The listing builds one solid part. Answer for the finished solid, in the listing's coordinates (mm). Face numbers are marked on the shaded views. A direction names the side the tool comes from. Coordinates: 2 decimals unless noted, no trailing zeros. Order: outer loops, then holes, each group sorted by start corner. A loop starts at its lowest first (then second) coordinate and runs counter-clockwise, first axis right, second up. Notation, with made-up numbers: (18, 43.5) -> (42, 43.5) arc R15 ccw to (42, 52.5) -> close; hole circle Ø1 at (41, -29.5). An arc over 180 degrees is marked (long way). Put each result on its own line as item: value. Start each with the question number.
```python
from build123d import *

# Parameters (mm, degrees)
SKETCH1_R           = 27
SKETCH1_R_2         = 8.8
BOSS_EXTRUDE1_DEPTH = 6.2
BOSS_EXTRUDE2_START = 2
SKETCH2_R           = 32.5
SKETCH2_R_2         = 8.8
BOSS_EXTRUDE2_DEPTH = 2
SKETCH3_W           = 5
SKETCH3_H           = 4.39677325
SKETCH3_W_2         = 4.39677325
SKETCH3_H_2         = 5
BOSS_EXTRUDE3_DEPTH = 6.2
BOSS_EXTRUDE4_DEPTH = 6.2


with BuildPart() as part:
    # Sketch1 → Boss-Extrude1 (new body)
    with BuildSketch(Plane(origin=(0, 0, 0), x_dir=(1, 0, 0), z_dir=(0, 1, 0))):
        with Locations(Location((0, 0, 0), (0, 0, 90))):
            Circle(SKETCH1_R)
        with Locations(Location((0, 0, 0), (0, 0, 90))):
            Circle(SKETCH1_R_2, mode=Mode.SUBTRACT)
        with BuildLine():
            Line((-17.5, -17.360083525), (-13.240365112, -13.134505385))
            ThreePointArc((-13.240365112, -13.134505385), (-17.20219229, -7.204656856), (-18.648686612, -0.221331548))
            Line((-18.648686612, -0.221331548), (-17.148571199, -0.221372599))
            ThreePointArc((-17.148571199, -0.221372599), (-15.815189186, -6.633422269), (-12.175456389, -12.07811085))
            Line((-12.175456389, -12.07811085), (-7.915821501, -7.85253271))
            ThreePointArc((-7.915821501, -7.85253271), (0, 11.15), (7.915821501, -7.85253271))
            Line((7.915821501, -7.85253271), (12.175456389, -12.07811085))
            ThreePointArc((12.175456389, -12.07811085), (15.815189186, -6.633422269), (17.148571199, -0.221372599))
            Line((17.148571199, -0.221372599), (18.648686612, -0.221331548))
            ThreePointArc((18.648686612, -0.221331548), (17.20219229, -7.204656856), (13.240365112, -13.134505385))
            Line((13.240365112, -13.134505385), (17.5, -17.360083525))
            ThreePointArc((17.5, -17.360083525), (0, 24.65), (-17.5, -17.360083525))
        make_face(mode=Mode.SUBTRACT)
    extrude(amount=BOSS_EXTRUDE1_DEPTH)

    # Sketch2 → Boss-Extrude2 (add)
    with BuildSketch(Plane.XZ.offset(BOSS_EXTRUDE2_START)):
        with Locations(Location((0, 0, 0), (0, 0, 270))):
            Circle(SKETCH2_R)
        with Locations(Location((0, 0, 0), (0, 0, 270))):
            Circle(SKETCH2_R_2, mode=Mode.SUBTRACT)
    extrude(amount=-BOSS_EXTRUDE2_DEPTH)

    # Sketch3 → Boss-Extrude3 (add)
    with BuildSketch(Plane(origin=(0, 0, 0), x_dir=(1, 0, 0), z_dir=(0, 1, 0))):
        with Locations((0, 27.601613375)):
            Rectangle(SKETCH3_W, SKETCH3_H)
        with Locations((27.601613375, 0)):
            Rectangle(SKETCH3_W_2, SKETCH3_H_2)
        with Locations((0, -27.601613375)):
            Rectangle(SKETCH3_W, SKETCH3_H)
        with Locations((-27.601613375, 0)):
            Rectangle(SKETCH3_W_2, SKETCH3_H_2)
    extrude(amount=BOSS_EXTRUDE3_DEPTH)

    # Sketch5 → Boss-Extrude4 (add)
    with BuildSketch(Plane(origin=(0, 0, 0), x_dir=(1, 0, 0), z_dir=(0, 1, 0))):
        with BuildLine():
            Line((-18.97760125, -15.731279376), (-13.203483223, -10.944886057))
            ThreePointArc((-13.203483223, -10.944886057), (-12.702113744, -11.522968647), (-12.175456389, -12.07811085))
            Line((-12.175456389, -12.07811085), (-17.733930638, -18.204578298))
            Line((-17.733930638, -18.204578298), (-18.97760125, -15.731279376))
        make_face()
    boss_extrude4 = extrude(amount=BOSS_EXTRUDE4_DEPTH)

    # Mirror2: Boss-Extrude4 across plane
    add(boss_extrude4.mirror(Plane(origin=(0, 0, 0), x_dir=(0, 0, 1), z_dir=(1, 0, 0))))


solid = part.part
```
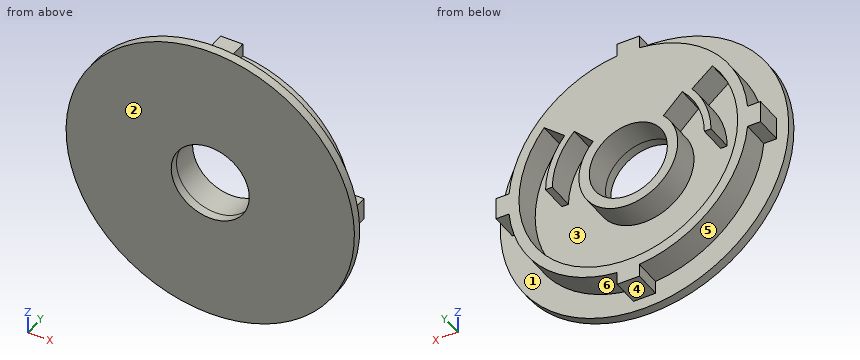
(1) The part is cut by section A-A on x = 0. Determine the outline of the cut face in (y, z), plus the area to 4 significant figures.
(2) Each of these flat-tipped pins is pushed along its axis until it touches: P1, Ø0.9, axis at y = 3.5, z = -28, coming from the +X side; P2, Ø1.5, axis at x = 1, y = 4, coming from the -Z side; P3, Ø1.5, axis at x = -1, y = 3, coming from the +Z side. Where does it stop, or does it pass through?
(3) The part is cut by section B-B on y = 1.5. Count the separate pieces of the cut face and the enclosed holes in it, plus the area to 3 significant figures.
(4) A tool of negligible diameter and unlimited length cuts with its end or side. For the marked faces 1 and 2, from which of +Z, -Z, +X, -X, +Y, -Y can it reach the whole face along a straight path? Write none if from no direction.
(5) For a pull along X with two mould halves and no side action, classify the marked faces 3, 4, 5 and 6 as released by +X, released by -X, zero draft, split by the parting line, or undercut.
(6) Find the intervals of material crossed by L1, parallel to Z at x = 0, y = 5; L2, parallel to X at y = 2, z = 0; L3, parallel to Z at x = 9, y = 5, in increasing order.
(7) The part is cut by section C-C on z = 14. Determine the outline of the cut face in (x, y).
Worked out:
1. outline: (-2, -32.5) -> (0, -32.5) -> (0, -29.8) -> (6.2, -29.8) -> (6.2, -24.65) -> (0, -24.65) -> (0, -11.15) -> (6.2, -11.15) -> (6.2, -8.8) -> (-2, -8.8) -> close; (-2, 8.8) -> (6.2, 8.8) -> (6.2, 29.8) -> (0, 29.8) -> (0, 32.5) -> (-2, 32.5) -> close
1. area: 271.5 mm2
2. P1: x = 2.5
2. P2: z = -29.8
2. P3: z = 29.8
3. separate pieces: 1
3. enclosed holes: 2
3. area: 1,030 mm2
4. face 1: +Y
4. face 2: +Z, -Z, +X, -X, -Y
5. face 3: undercut
5. face 4: zero draft
5. face 5: released by -X
5. face 6: released by +X
6. L1: -29.8 to -24.65, -11.15 to -8.8, 8.8 to 29.8
6. L2: -29.8 to -24.65, -11.15 to -8.8, 8.8 to 11.15, 24.65 to 29.8
6. L3: -25.46 to -22.95, -6.58 to 6.58, 8.93 to 25.46
7. outline: (-29.33, -2) -> (29.33, -2) -> (29.33, 0) -> (23.09, 0) -> (23.09, 6.2) -> (20.29, 6.2) -> (20.29, 0) -> (16.89, 0) -> (16.89, 6.2) -> (-16.89, 6.2) -> (-16.89, 0) -> (-20.29, 0) -> (-20.29, 6.2) -> (-23.09, 6.2) -> (-23.09, 0) -> (-29.33, 0) -> close
